Work out the finished part from the listing and answer in its coordinate system (mm). A direction names the side the tool comes from. Coordinates: 2 decimals unless noted, no trailing zeros. Order: outer loops, then holes, each group sorted by start corner. A loop starts at its lowest first (then second) coordinate and runs counter-clockwise, first axis right, second up. Notation, with made-up numbers: M 84.25,32 L 132.25,32 A16 cw 132.25,46 Z; hole C 60.25,75 d11. An arc over 180 degrees is marked long. Use a Markdown table: item, result.
from build123d import *

# Parameters (mm, degrees)
SKETCH1_W           = 315
SKETCH1_H           = 266
BOSS_EXTRUDE1_DEPTH = 100
SHELL1_START        = -154.5
SHELL1_OUTLINE_W    = 92
SHELL1_OUTLINE_H    = 260
SHELL1_DEPTH        = 309
SKETCH2_W           = 309
SKETCH2_H           = 260
CUT_EXTRUDE1_DEPTH  = 3
SKETCH5_W           = 50
SKETCH5_H           = 35
CUT_EXTRUDE3_DEPTH  = 2


# Read off the part's stored shape, not the designer's step: Shell1
with BuildPart() as part:
    # Sketch1 → Boss-Extrude1 (new body)
    with BuildSketch(Plane(origin=(0, 0, 0), x_dir=(1, 0, 0), z_dir=(0, 1, 0))):
        Rectangle(SKETCH1_W, SKETCH1_H)
    extrude(amount=BOSS_EXTRUDE1_DEPTH)

    # Shell1 outline → Shell1 (cut)
    with BuildSketch(Plane.YZ.offset(SHELL1_START)):
        with Locations((51, 0)):
            Rectangle(SHELL1_OUTLINE_W, SHELL1_OUTLINE_H)
    extrude(amount=SHELL1_DEPTH, mode=Mode.SUBTRACT)

    # Sketch2 → Cut-Extrude1 (cut)
    with BuildSketch(Plane(origin=(0, 100, 0), x_dir=(1, 0, 0), z_dir=(0, 1, 0))):
        Rectangle(SKETCH2_W, SKETCH2_H)
    extrude(amount=-CUT_EXTRUDE1_DEPTH, mode=Mode.SUBTRACT)

    # Sketch5 → Cut-Extrude3 (cut)
    with BuildSketch(Plane.XY.offset(-130)):
        with Locations((-77.25, 82.5)):
            Rectangle(SKETCH5_W, SKETCH5_H)
    cut_extrude3 = extrude(amount=-CUT_EXTRUDE3_DEPTH, mode=Mode.SUBTRACT)

    # Mirror1: Cut-Extrude3 across plane
    add(cut_extrude3.mirror(Plane(origin=(0, 0, 0), x_dir=(0, 0, 1), z_dir=(1, 0, 0))), mode=Mode.SUBTRACT)


solid = part.part
(1) Determine the mould class of faces 3 (the flat face through (-154.5, 53, 2)), 4 (the flat face through (-157.5, 49, 2)), 5 (the flat face through (-2, 49, -133)) for opening direction X: pulls with the +X half, pulls with the -X half, needs draft (parallel to the pull), parting line crosses it, or undercut.
Conclusion:
| item | result |
|---|---|
| face 3 | undercut |
| face 4 | pulls with the -X half |
| face 5 | needs draft |
(2) A cutting plane is placed at A-A (y = 26). Determine the outline of the cut face in (x, z).
Conclusion:
| item | result |
|---|---|
| outline | M -157.5,-133 L 157.5,-133 L 157.5,133 L -157.5,133 Z; hole M -154.5,-130 L 154.5,-130 L 154.5,130 L -154.5,130 Z |
(3) A cutting plane is placed at C-C (z = 97.5). Determine the outline of the cut face in (x, y).
Conclusion:
| item | result |
|---|---|
| outline | M -157.5,0 L 157.5,0 L 157.5,100 L 154.5,100 L 154.5,5 L -154.5,5 L -154.5,100 L -157.5,100 Z |
(4) A cutting plane is placed at D-D (y = 78). Determine the outline of the cut face in (x, z), then the cut area to 3 significant figures.
Conclusion:
| item | result |
|---|---|
| outline | M -157.5,-133 L 157.5,-133 L 157.5,133 L -157.5,133 Z; hole M -154.5,-130 L -102.25,-130 L -102.25,-132 L -52.25,-132 L -52.25,-130 L 52.25,-130 L 52.25,-132 L 102.25,-132 L 102.25,-130 L 154.5,-130 L 154.5,130 L -154.5,130 Z |
| area | 3,250 mm2 |
(5) A cutting plane is placed at B-B (x = -35.5). Determine the outline of the cut face in (y, z), then the cut area to 3 significant figures.
Conclusion:
| item | result |
|---|---|
| outline | M 0,-133 L 100,-133 L 100,-130 L 5,-130 L 5,130 L 100,130 L 100,133 L 0,133 Z |
| area | 1,900 mm2 |
(6) Straight lines are drawn through the part: L1, parallel to X at y = 55, z = -37; L2, parallel to Z at x = -63.5, y = 92; L3, parallel to Z at x = 7, y = 74. For each, find the intervals that lie inside material, in ascending order.
Conclusion:
| item | result |
|---|---|
| L1 | -157.5 to -154.5, 154.5 to 157.5 |
| L2 | -133 to -132, 130 to 133 |
| L3 | -133 to -130, 130 to 133 |
(7) Which of the six approach directions +Z, -Z, +X, -X, +Y, -Y give full straight-line access (tool end or side, diameter ignored) to faces 1 (the flat face through (-2, 53, 130)), 2 (the flat face through (-2, 0, -2))?
Conclusion:
| item | result |
|---|---|
| face 1 | +Y |
| face 2 | +Z, -Z, +X, -X, -Y |
(8) Given P1, Ø3, axis at x = 19, z = 0, coming from the +Y side; P2, Ø0.6, axis at x = -70.5, z = -130.5, coming from the +Y side, each flat-ended and moving along its own axis, determine where each tip first touches the part or whether it passes through.
Conclusion:
| item | result |
|---|---|
| P1 | y = 5 |
| P2 | y = 65 |
